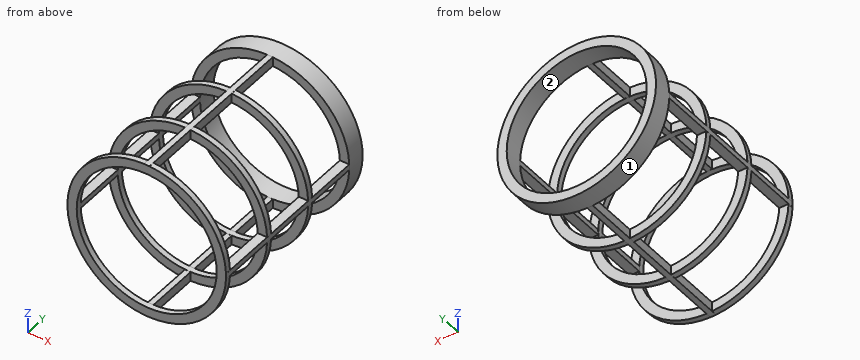
```python
from build123d import *

# Parameters (mm, degrees)
SKETCH1_W           = 6.35
SKETCH1_H           = 12.7
BOSS_EXTRUDE1_DEPTH = 1.905
CIRPATTERN1_COUNT   = 2
CIRPATTERN1_ANGLE   = 90
SKETCH2_R           = 53.975
SKETCH2_R_2         = 47.625
BOSS_EXTRUDE2_DEPTH = 3.81
LPATTERN1_COUNT     = 3
LPATTERN1_PITCH     = 39.15833418
SKETCH4_R           = 60.96
CUT_EXTRUDE1_DEPTH  = 66.04


with BuildPart() as part:
    # Sketch1 → Revolve6 (revolve)
    with BuildSketch(Plane(origin=(0, 0, 0), x_dir=(0, 0, -1), z_dir=(1, 0, 0))):
        with Locations((3.175, -6.35)):
            Rectangle(SKETCH1_W, SKETCH1_H)
    revolve(axis=Axis((0, -130.175, -53.975), (0, -1, 0)))

    # Sketch1_6 → Boss-Extrude1 (add, symmetric)
    with BuildSketch(Plane(origin=(0, 0, 0), x_dir=(0, 0, -1), z_dir=(1, 0, 0))):
        with BuildLine():
            ThreePointArc((6.35, -130.175), (53.975, -177.8), (101.6, -130.175))
            Line((101.6, -130.175), (101.6, -12.7))
            Line((101.6, -12.7), (107.95, -12.7))
            Line((107.95, -12.7), (107.95, -130.175))
            ThreePointArc((107.95, -130.175), (53.975, -184.15), (0, -130.175))
            Line((0, -130.175), (0, -12.7))
            Line((0, -12.7), (6.35, -12.7))
            Line((6.35, -12.7), (6.35, -130.175))
        make_face()
    boss_extrude1 = extrude(amount=BOSS_EXTRUDE1_DEPTH, both=True)

    # CirPattern1: Boss-Extrude1 ×2 about axis
    cirpattern1_axis = Axis((0, 0, -53.975), (0, -1, 0))
    for i in range(1, CIRPATTERN1_COUNT):
        add(boss_extrude1.rotate(cirpattern1_axis, i * CIRPATTERN1_ANGLE / (CIRPATTERN1_COUNT - 1)))

    # Sketch2 → Boss-Extrude2 (add)
    with BuildSketch(Plane(origin=(0, -130.175, 0), x_dir=(-1, 0, 0), z_dir=(0, -1, 0))):
        with Locations(Location((0, 53.975, 0), (0, 0, 270))):
            Circle(SKETCH2_R)
        with Locations(Location((0, 53.975, 0), (0, 0, 270))):
            Circle(SKETCH2_R_2, mode=Mode.SUBTRACT)
    boss_extrude2 = extrude(amount=-BOSS_EXTRUDE2_DEPTH)

    # LPattern1: Boss-Extrude2 ×3
    with Locations(*[(0, i * LPATTERN1_PITCH, 0) for i in range(1, LPATTERN1_COUNT)]):
        add(boss_extrude2)

    # Sketch4 → Cut-Extrude1 (cut)
    with BuildSketch(Plane.XZ.offset(130.175)):
        with Locations((0, -53.975)):
            Circle(SKETCH4_R)
    extrude(amount=CUT_EXTRUDE1_DEPTH, mode=Mode.SUBTRACT)


solid = part.part
```
Design review of the part built by this model. Coordinates are the model's own, in mm. Face numbers are marked on the shaded views. Coordinates: 2 decimals unless noted, no trailing zeros. Order: outer loops, then holes, each group sorted by start corner. A loop starts at its lowest first (then second) coordinate and runs counter-clockwise, first axis right, second up. Notation, with made-up numbers: M 33,28 L 92,28 A34 cw 92,62 Z; hole C -37.75,5.25 d3. An arc over 180 degrees is marked long. Answer as a JSON object with one key per item and string values. Group by question number.
1) Mouldability with a two-part tool opening along X and no side actions: class the marked faces 1 and 2 as pulls with the +X half, pulls with the -X half, needs draft (parallel to the pull), parting line crosses it, or undercut.
2) Add section B-B, the plane y = -81.5. Write out the cut boundary in (x, z) (3 decimals).
3) Add section A-A, the plane z = -67.5. Count the separate pieces of the cut face and the enclosed holes in it, then the cut area to 3 significant figures.
4) Wall thickness on L1, parallel to Y at x = 20, z = -5 (3 decimals); L2, parallel to Z at x = 1, y = -40: over which ranges is each line inside the solid? List them lowest first.
5) For pin 1 (6 mm diameter, centred on x = -41.5, z = -35, fed in from +Y); pin 2 (1 mm diameter, centred on x = -21.5, y = -90.5, fed in from -Z); pin 3 (3 mm diameter, centred on y = -91.5, z = -105, fed in from +X), all flat-tipped, find the tip position at first contact; note any pin that passes through.
Computed values:
{
 "1": {"face 1": "parting line crosses it", "face 2": "undercut"},
 "2": {"outline": "M -53.975,-55.88 L -47.625,-55.88 L -47.625,-52.07 L -53.975,-52.07 Z; M -1.905,-107.95 L 1.905,-107.95 L 1.905,-101.6 L -1.905,-101.6 Z; M -1.905,-6.35 L 1.905,-6.35 L 1.905,0 L -1.905,0 Z; M 47.625,-55.88 L 53.975,-55.88 L 53.975,-52.07 L 47.625,-52.07 Z"},
 "3": {"separate pieces": "8", "enclosed holes": "0", "area": "318 mm^2"},
 "4": {"L1": "y = -130.175 to -126.365, -91.017 to -87.207, -51.858 to -48.048, -12.7 to 0", "L2": "z = -107.95 to -101.6, -6.35 to 0"},
 "5": {"pin 1": "stops at y = 0", "pin 2": "stops at z = -103.7", "pin 3": "stops at x = 21.28"}
}
